from build123d import *

# Parameters (mm, degrees)
F1_DEPTH = 63.5
F0_W     = 25.4
F0_H     = 16.51
F2_DEPTH = 25.4
F3_DEPTH = 15.875
F5_R     = 5.08


with BuildPart() as f1:
    # F0 (on Front) → F1 (new body, symmetric)
    with BuildSketch(Plane.XZ):
        Polygon((-41.275, -9.525), (41.275, -9.525), (41.275, 9.525), (24.765, 9.525), (-41.275, 9.525), align=None)
    extrude(amount=F1_DEPTH, both=True)

    # F0 (on Front) → F2 (join, symmetric)
    with BuildSketch(Plane.XZ):
        with BuildLine():
            Line((24.765, 9.525), (41.275, 9.525))
            Line((41.275, 9.525), (41.275, 27.0002))
            ThreePointArc((41.275, 27.0002), (45.9246798487, 38.2255201513), (57.15, 42.8752))
            Line((57.15, 42.8752), (71.6676590706, 42.8752))
            Line((71.6676590706, 42.8752), (71.6676590706, 59.3852))
            Line((71.6676590706, 59.3852), (57.15, 59.3852))
            add(Edge.make_bspline(
                [(55.4911539535, 59.3426868369), (56.0411228755, 59.3576141574), (56.5940666192, 59.3717855904), (57.15, 59.3852)],
                knots=[109.5705582986, 109.5705582986, 109.5705582986, 109.5705582986, 110.3336764956, 110.3336764956, 110.3336764956, 110.3336764956], degree=3))
            ThreePointArc((55.4911539535, 59.3426868369), (33.6711802446, 49.3056533218), (24.765, 27.0002))
            Line((24.765, 27.0002), (24.765, 9.525))
        make_face()
        with Locations((84.3676590706, 51.1302)):
            Rectangle(F0_W, F0_H)
    extrude(amount=F2_DEPTH, both=True)

    # F0 (on Front) → F3 (join)
    with BuildSketch(Plane.XZ):
        with BuildLine():
            add(Edge.make_bspline(
                [(-41.275, 9.525), (-41.1119862011, 39.4727109484), (-23.4748595098, 57.1993821099), (55.4911539535, 59.3426868369)],
                knots=[0, 0, 0, 0, 109.5705582986, 109.5705582986, 109.5705582986, 109.5705582986], degree=3))
            Line((-41.275, 9.525), (24.765, 9.525))
            Line((24.765, 9.525), (24.765, 27.0002))
            ThreePointArc((24.765, 27.0002), (33.6711802446, 49.3056533218), (55.4911539535, 59.3426868369))
        make_face()
    extrude(amount=F3_DEPTH)

    # F0 (on Front) → F4 (revolve)
    with BuildSketch(Plane.XZ):
        Polygon((97.0676590706, 59.3852), (97.0676590706, 42.8752), (97.0676590706, 38.2255201513), (122.4676590706, 38.2255201513), (122.4676590706, 66.675), (97.0676590706, 66.675), align=None)
    revolve(axis=Axis((97.0676590706, 0, 52.4502600757), (0, 0, 1)))

    # F5
    f5_edges = [f1.edges().sort_by_distance(p)[0] for p in [
        (41.275, -63.5, 0),
        (-41.275, -63.5, 0),
        (41.275, 63.5, 0),
        (-41.275, 63.5, 0),
    ]]
    fillet(f5_edges, radius=F5_R)


solid = f1.part
The model under review builds one solid part; all positions refer to its coordinate system, in mm. A direction names the side the tool comes from. Round coordinates to 2 decimals unless told otherwise and drop trailing zeros. Write each loop counter-clockwise with the first axis right and the second up, starting at its lowest first coordinate (ties: lowest second). Pieces come first, ordered by that corner, then holes. Notation, with made-up numbers: M 62.5,83 L 107.5,83 A14 ccw 107.5,95 Z; hole C 67,31.5 d3. An arc over 180 degrees is marked long. Use a Markdown table: item, result. Add a question column.
Q1. Insertion check: pin 1 (8.5 mm diameter, centred on y = 11, z = 14, fed in from -X) (3 decimals); pin 2 (15 mm diameter, centred on x = 1.5, z = 28.5, fed in from +Y); pin 3 (1.5 mm diameter, centred on y = 14, z = 7.5, fed in from +X) (3 decimals). Each pin has a flat end and moves straight along its axis. Give the tip position at first contact, or say it passes through.
Q2. We need section B-B, the plane y = 48.5. State the section outline as (x, z) points (3 decimals).
Q3. To check wall thickness, follow line 1 (Z direction, x = 97.5, y = 23) (3 decimals); line 2 (Z direction, x = 2, y = -24.5) (3 decimals); line 3 (Y direction, x = -1, z = 52.5) (3 decimals). State the ranges of each line that lie inside material, in increasing order.
Q4. We need section A-A, the plane z = -1. State the section outline as (x, y) points (3 decimals), plus the area to 3 significant figures.
Q5. The part is to be moulded in two halves that separate along X. For faces 1 (the face through (24.765, -21, 18)), 2 (the face through (68, 0, 42.875)), 3 (the face through (-1, -1, -9.525)), say which applies: pulls with the +X half, pulls with the -X half, needs draft (parallel to the pull), parting line crosses it, or undercut.
Q6. Machinability: for faces 4 (the face through (97, 0, 38.226)), 5 (the face through (69, 0, 59.385)), 6 (the face through (45.8, -0.4, 38.1)), which of the approach directions +Z, -Z, +X, -X, +Y, -Y give a long, thin tool a straight path to every point of the face, cutting with its end or side? Answer none if there is none.
Findings below:
| question | item | result |
|---|---|---|
| 1 | pin 1 | stops at x = 24.765 |
| 1 | pin 2 | stops at y = 0 |
| 1 | pin 3 | stops at x = 41.275 |
| 2 | outline | M -41.275,-9.525 L 41.275,-9.525 L 41.275,9.525 L -41.275,9.525 Z |
| 3 | line 1 | z = 38.226 to 66.675 |
| 3 | line 2 | z = -9.525 to 9.525 |
| 3 | line 3 | y = -15.875 to 0 |
| 4 | outline | M -41.275,-58.42 A5.08 ccw -36.195,-63.5 L 36.195,-63.5 A5.08 ccw 41.275,-58.42 L 41.275,58.42 A5.08 ccw 36.195,63.5 L -36.195,63.5 A5.08 ccw -41.275,58.42 Z |
| 4 | area | 10,500 mm² |
| 5 | face 1 | pulls with the -X half |
| 5 | face 2 | undercut |
| 5 | face 3 | needs draft |
| 6 | face 4 | -Z, +X, +Y, -Y |
| 6 | face 5 | +Z, -X |
| 6 | face 6 | -Z, +Y, -Y |
